from build123d import *

# Parameters (mm, degrees)
ESQUISSE1_R             = 3
BOSS_EXTRU_3_DEPTH      = 6
ENL_V_MAT_EXTRU_2_DEPTH = 3
ESQUISSE5_R             = 2
ESQUISSE5_R_2           = 3
ENL_V_MAT_EXTRU_3_DEPTH = 3


with BuildPart() as part:
    # Esquisse1 → Boss.-Extru.3 (new body)
    with BuildSketch(Plane.XY):
        with BuildLine():
            Line((7.993323256, 75.345483427), (102.993323256, 75.345483427))
            ThreePointArc((102.993323256, 75.345483427), (109.710837677, 72.562997848), (112.493323256, 65.845483427))
            Line((112.493323256, 65.845483427), (112.493323256, 5.845483427))
            ThreePointArc((112.493323256, 5.845483427), (109.710837677, -0.872030995), (102.993323256, -3.654516573))
            Line((102.993323256, -3.654516573), (7.993323256, -3.654516573))
            ThreePointArc((7.993323256, -3.654516573), (1.275808835, -0.872030995), (-1.506676744, 5.845483427))
            Line((-1.506676744, 5.845483427), (-1.506676744, 65.845483427))
            ThreePointArc((-1.506676744, 65.845483427), (1.275808835, 72.562997848), (7.993323256, 75.345483427))
        make_face()
        with Locations((107.493323256, 65.845483427)):
            Circle(ESQUISSE1_R, mode=Mode.SUBTRACT)
        with Locations((107.493323256, 25.845483427)):
            Circle(ESQUISSE1_R, mode=Mode.SUBTRACT)
        with Locations((3.493323256, 65.845483427)):
            Circle(ESQUISSE1_R, mode=Mode.SUBTRACT)
        with Locations((3.493323256, 25.845483427)):
            Circle(ESQUISSE1_R, mode=Mode.SUBTRACT)
    extrude(amount=BOSS_EXTRU_3_DEPTH)

    # Esquisse3 → Enlèv. mat.-Extru.2 (cut)
    with BuildSketch(Plane.XY.offset(6)):
        with BuildLine():
            Line((4.493323256, 74.345483427), (106.493323256, 74.345483427))
            ThreePointArc((106.493323256, 74.345483427), (110.028857162, 72.881017333), (111.493323256, 69.345483427))
            Line((111.493323256, 69.345483427), (111.493323256, 2.345483427))
            ThreePointArc((111.493323256, 2.345483427), (110.028857162, -1.190050479), (106.493323256, -2.654516573))
            Line((106.493323256, -2.654516573), (4.493323256, -2.654516573))
            ThreePointArc((4.493323256, -2.654516573), (0.95778935, -1.190050479), (-0.506676744, 2.345483427))
            Line((-0.506676744, 2.345483427), (-0.506676744, 69.345483427))
            ThreePointArc((-0.506676744, 69.345483427), (0.95778935, 72.881017333), (4.493323256, 74.345483427))
        make_face()
    extrude(amount=-ENL_V_MAT_EXTRU_2_DEPTH, mode=Mode.SUBTRACT)

    # Esquisse5 → Enlèv. mat.-Extru.3 (cut)
    with BuildSketch(Plane.XY.offset(3)):
        with Locations((10.993323256, 70.345483427)):
            Circle(ESQUISSE5_R)
        with Locations((99.993323256, 70.345483427)):
            Circle(ESQUISSE5_R)
        with Locations((10.993323256, 1.345483427)):
            Circle(ESQUISSE5_R)
        with Locations((99.993323256, 1.345483427)):
            Circle(ESQUISSE5_R)
        with Locations((41.993323256, 8.845483427)):
            Circle(ESQUISSE5_R_2)
        with Locations((71.493323256, 8.845483427)):
            Circle(ESQUISSE5_R_2)
        with Locations((36.493323256, 67.473019046)):
            Circle(ESQUISSE5_R)
        with Locations((34.493323256, 19.473019046)):
            Circle(ESQUISSE5_R)
        with Locations((86.993323256, 51.973019046)):
            Circle(ESQUISSE5_R)
        with Locations((86.993323256, 24.973019046)):
            Circle(ESQUISSE5_R)
    extrude(amount=-ENL_V_MAT_EXTRU_3_DEPTH, mode=Mode.SUBTRACT)


solid = part.part
CAD build for the part. Positions are in the model's coordinates, mm. Give positions to 0.01 mm unless a question says otherwise; leave off trailing zeros. Write each loop counter-clockwise with the first axis right and the second up, starting at its lowest first coordinate (ties: lowest second). Pieces come first, ordered by that corner, then holes. Notation, with made-up numbers: (21, -2.5) - (77, -2.5) arc R23 cw to (77, 22.5) - close; hole circle Ø9 at (40.25, -33.5). An arc over 180 degrees is marked (long way). Answer as CSV lines item,"result".
Q1. Band-saw the part on C-C (y = 46.5). Give the cut face in (x, z).
Result set:
outline,"(-1.51, 0) - (112.49, 0) - (112.49, 6) - (111.49, 6) - (111.49, 3) - (-0.51, 3) - (-0.51, 6) - (-1.51, 6) - close"
Q2. Flat gauge pins, fed straight in: pin 1 Ø5 at (x, y) = (71.49, 8.85) entering from -Z; pin 2 Ø6.5 at (x, y) = (34.49, 19.47) entering from +Z. Where does each tip first touch, or does it go through?
Result set:
pin 1,"through"
pin 2,"z = 3"
Q3. Pull direction Y, two halves, no side cores. Call faces 1 (the face through (36.06, 65.52, 1.52)), 2 (the face through (12.9, 1.95, 1.52)), 3 (the face through (1.35, -0.945, 2.291)), 4 (the face through (109.637, 72.636, 2.291)): released by +Y, released by -Y, zero draft, split by the parting line, or undercut.
Result set:
face 1,"undercut"
face 2,"undercut"
face 3,"released by -Y"
face 4,"released by +Y"
Q4. Drill centre lines: line 1 (X direction, y = 57.5, z = 3.3); line 2 (Y direction, x = 45.5, z = 3.8); line 3 (X direction, y = 8, z = 2.45). Where is each one in solid material? Low to high. Write a range as from..to.
Result set:
line 1,"-1.51..-0.51, 111.49..112.49"
line 2,"-3.65..-2.65, 74.35..75.35"
line 3,"-1.51..39.11, 44.87..68.61, 74.37..112.49"
Q5. Band-saw the part on A-A (z = 4.25). Give the cut face in (x, y), and give its area (3 significant figures).
Result set:
outline,"(-1.51, 5.85) arc R9.5 ccw to (-0.42, 1.44) arc R5 cw to (-0.51, 2.35) - (-0.51, 69.35) arc R5 cw to (-0.42, 70.25) arc R9.5 ccw to (-1.51, 65.85) - close; (3.59, -2.57) arc R9.5 ccw to (7.99, -3.65) - (102.99, -3.65) arc R9.5 ccw to (107.4, -2.57) arc R5 cw to (106.49, -2.65) - (4.49, -2.65) arc R5 cw to start; (3.59, 74.26) arc R5 cw to (4.49, 74.35) - (106.49, 74.35) arc R5 cw to (107.4, 74.26) arc R9.5 ccw to (102.99, 75.35) - (7.99, 75.35) arc R9.5 ccw to start; (111.41, 1.44) arc R9.5 ccw to (112.49, 5.85) - (112.49, 65.85) arc R9.5 ccw to (111.41, 70.25) arc R5 cw to (111.49, 69.35) - (111.49, 2.35) arc R5 cw to start"
area,"333 mm²"
Q6. Band-saw the part on B-B (x = 22.5). Give the cut face in (y, z), and give its area (3 significant figures).
Result set:
outline,"(-3.65, 0) - (75.35, 0) - (75.35, 6) - (74.35, 6) - (74.35, 3) - (-2.65, 3) - (-2.65, 6) - (-3.65, 6) - close"
area,"243 mm²"
